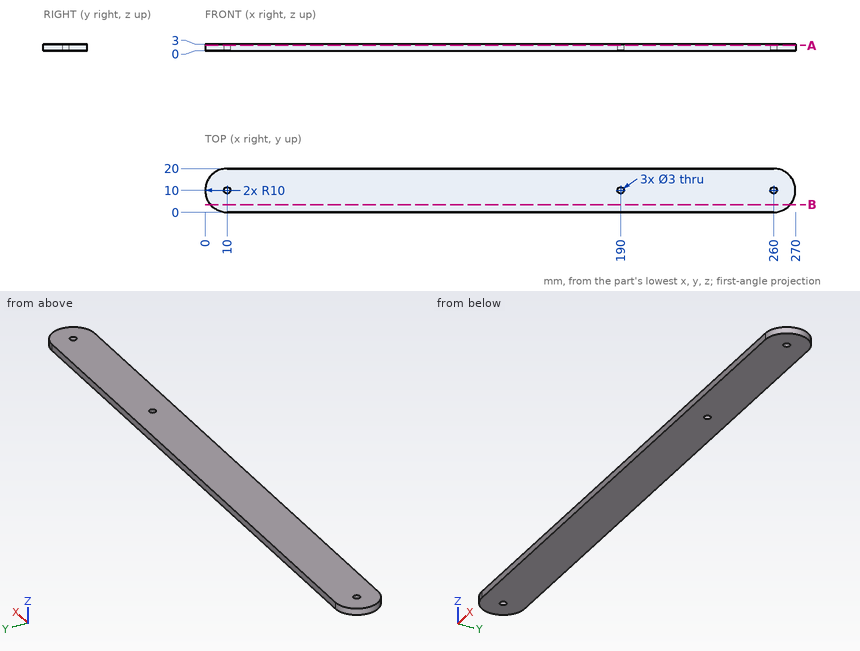
Answer from the drawing. Dimensions are ordinates in mm from the lowest x, y and z of the part. Coordinates: 2 decimals unless noted, no trailing zeros. Loops run counter-clockwise (first coordinate to the right, second up) from the corner with the lowest first, then second, coordinate; pieces in that order, holes last.
Q1. The part is cut by section B-B on y = 3.5. Write down the section's boundary in (x, z).
Q2. Consider probe 1 along X at (y, z) = (10, 1.8); probe 2 along Y at (x, z) = (260, 0.8); probe 3 along X at (y, z) = (9.25, 0.4). Determine where each line is inside the solid, lowest interval first.
Q3. The part is cut by section A-A on z = 2.35. Write down the section's boundary in (x, y), and give its area (3 significant figures).
Results below:
1. outline: (2.4, 0) - (267.6, 0) - (267.6, 3) - (2.4, 3) - close
2. probe 1: x = 0 to 8.5, 11.5 to 188.5, 191.5 to 258.5, 261.5 to 270
2. probe 2: y = 0 to 8.5, 11.5 to 20
2. probe 3: x = 0.03 to 8.7, 11.3 to 188.7, 191.3 to 258.7, 261.3 to 269.97
3. outline: (10, 0) - (260, 0) arc R10 ccw to (260, 20) - (10, 20) arc R10 ccw to start; hole circle Ø3 at (10, 10); hole circle Ø3 at (190, 10); hole circle Ø3 at (260, 10)
3. area: 5,290 mm2
